```python
from build123d import *

# Parameters (mm, degrees)
EXTRUDE1_DEPTH             = 900
EXTRUDE2_REACH             = 902.087
SKETCH2_R                  = 2.25
SKETCH_R                   = 3
SKETCH_R_2                 = 2.25
EXTRUDE4_DEPTH             = 2.3
CHAMFER1_SIZE              = 0.2
LPATTERN1_COUNT            = 22
LPATTERN1_PITCH            = 40
CHAMFER1_OF_LPATTERN1_SIZE = 0.2


with BuildPart() as part:
    # Sketch1 → Extrude1 (new body)
    with BuildSketch(Plane.XY):
        with BuildLine():
            Line((-7.3, -5), (7.3, -5))
            Line((7.3, -5), (7.5, -4.8))
            Line((7.5, -4.8), (7.5, 2.706274607))
            ThreePointArc((7.5, 2.706274607), (7.091294745, 2.882570681), (6.840065792, 3.25))
            Line((6.840065792, 3.25), (6.340065792, 3.25))
            Line((6.340065792, 3.25), (6.340065792, 3.75))
            Line((6.340065792, 3.75), (6.840065792, 3.75))
            ThreePointArc((6.840065792, 3.75), (7.091294745, 4.117429319), (7.5, 4.293725393))
            Line((7.5, 4.293725393), (7.5, 4.8))
            Line((7.5, 4.8), (7.3, 5))
            Line((7.3, 5), (-7.3, 5))
            Line((-7.3, 5), (-7.5, 4.8))
            Line((-7.5, 4.8), (-7.5, 4.293725393))
            ThreePointArc((-7.5, 4.293725393), (-7.091294745, 4.117429319), (-6.840065792, 3.75))
            Line((-6.840065792, 3.75), (-6.340065792, 3.75))
            Line((-6.340065792, 3.75), (-6.340065792, 3.25))
            Line((-6.340065792, 3.25), (-6.840065792, 3.25))
            ThreePointArc((-6.840065792, 3.25), (-7.091294745, 2.882570681), (-7.5, 2.706274607))
            Line((-7.5, 2.706274607), (-7.5, -4.8))
            Line((-7.5, -4.8), (-7.3, -5))
        make_face()
    extrude(amount=EXTRUDE1_DEPTH)

    # Sketch2 → Extrude2 (cut, up to next)
    with BuildSketch(Plane(origin=(0, 5, 0), x_dir=(1, 0, 0), z_dir=(0, 1, 0)), mode=Mode.PRIVATE) as extrude2_sk1:
        with Locations(Location((0, -15, 0), (0, 0, 270))):
            Circle(SKETCH2_R)
    extrude2_tool1 = extrude(extrude2_sk1.sketch, amount=-EXTRUDE2_REACH, mode=Mode.PRIVATE) & part.part
    extrude2 = extrude2_tool1.solids().sort_by_distance((0, 5, 15))[0]
    add(extrude2, mode=Mode.SUBTRACT)

    # Sketch → Extrude4 (cut)
    with BuildSketch(Plane(origin=(0, 5, 0), x_dir=(1, 0, 0), z_dir=(0, 1, 0))):
        with Locations(Location((0, -15, 0), (0, 0, 270))):
            Circle(SKETCH_R)
        with Locations(Location((0, -15, 0), (0, 0, 270))):
            Circle(SKETCH_R_2, mode=Mode.SUBTRACT)
    extrude4 = extrude(amount=-EXTRUDE4_DEPTH, mode=Mode.SUBTRACT)

    # Chamfer1
    chamfer1_edges = [part.edges().sort_by_distance(p)[0] for p in [
        (0, -5, 12.75),
        (0, 5, 12),
    ]]
    chamfer(chamfer1_edges, length=CHAMFER1_SIZE)

    # LPattern1: Extrude2, Extrude4 ×22
    with Locations(*[(0, 0, i * LPATTERN1_PITCH) for i in range(1, LPATTERN1_COUNT)]):
        add(extrude2, mode=Mode.SUBTRACT)
        add(extrude4, mode=Mode.SUBTRACT)

    # Chamfer1 of LPattern1
    chamfer1_of_lpattern1_edges = [part.edges().sort_by_distance(p)[0] for p in [
        (0, -5, 52.75),
        (0, 5, 52),
        (0, -5, 92.75),
        (0, 5, 92),
        (0, -5, 132.75),
        (0, 5, 132),
        (0, -5, 172.75),
        (0, 5, 172),
        (0, -5, 212.75),
        (0, 5, 212),
        (0, -5, 252.75),
        (0, 5, 252),
        (0, -5, 292.75),
        (0, 5, 292),
        (0, -5, 332.75),
        (0, 5, 332),
        (0, -5, 372.75),
        (0, 5, 372),
        (0, -5, 412.75),
        (0, 5, 412),
        (0, -5, 452.75),
        (0, 5, 452),
        (0, -5, 492.75),
        (0, 5, 492),
        (0, -5, 532.75),
        (0, 5, 532),
        (0, -5, 572.75),
        (0, 5, 572),
        (0, -5, 612.75),
        (0, 5, 612),
        (0, -5, 652.75),
        (0, 5, 652),
        (0, -5, 692.75),
        (0, 5, 692),
        (0, -5, 732.75),
        (0, 5, 732),
        (0, -5, 772.75),
        (0, 5, 772),
        (0, -5, 812.75),
        (0, 5, 812),
        (0, -5, 852.75),
        (0, 5, 852),
    ]]
    chamfer(chamfer1_of_lpattern1_edges, length=CHAMFER1_OF_LPATTERN1_SIZE)


solid = part.part
```
CAD build for the part. Positions are in the model's coordinates, mm. Coordinates: 2 decimals unless noted, no trailing zeros. Write each question's results on one line, items separated by ' | '. Start each with the question number.
Q1. Drill centre lines: probe 1 along X at (y, z) = (-2.5, 55); probe 2 along X at (y, z) = (3.95, 95); probe 3 along Y at (x, z) = (6.5, 57). Where is each one in solid material? Low to high. Write a range as from..to.
Q2. Flat gauge pins, fed straight in: P1, Ø5, axis at x = 0, z = 135, coming from the +Y side; P2, Ø6.5, axis at x = 0, z = 534.5, coming from the +Y side. Where does each tip first touch, or does it go through?
Q3. Cut at A-A (y = -2). Count the separate pieces of the cut face and the enclosed holes in it, then the cut area to 3 significant figures.
Found:
1) probe 1: -7.5..-2.25, 2.25..7.5 | probe 2: -6.94..-3, 3..6.94 | probe 3: -5..3.25, 3.75..5
2) P1: y = 2.7 | P2: y = 5
3) separate pieces: 1 | enclosed holes: 22 | area: 13,200 mm²
